Drawing for the job (mm, zero at the part's lowest x, y, z). A direction names the side the tool comes from. Give positions to 0.01 mm unless a question says otherwise; leave off trailing zeros. Order: outer loops, then holes, each group sorted by start corner. A loop starts at its lowest first (then second) coordinate and runs counter-clockwise, first axis right, second up. Notation, with made-up numbers: M 69.5,56.5 L 79.5,56.5 A23 cw 79.5,92.5 Z; hole C 4.5,35 d5. An arc over 180 degrees is marked long. Answer as a JSON object with one key per item and string values.
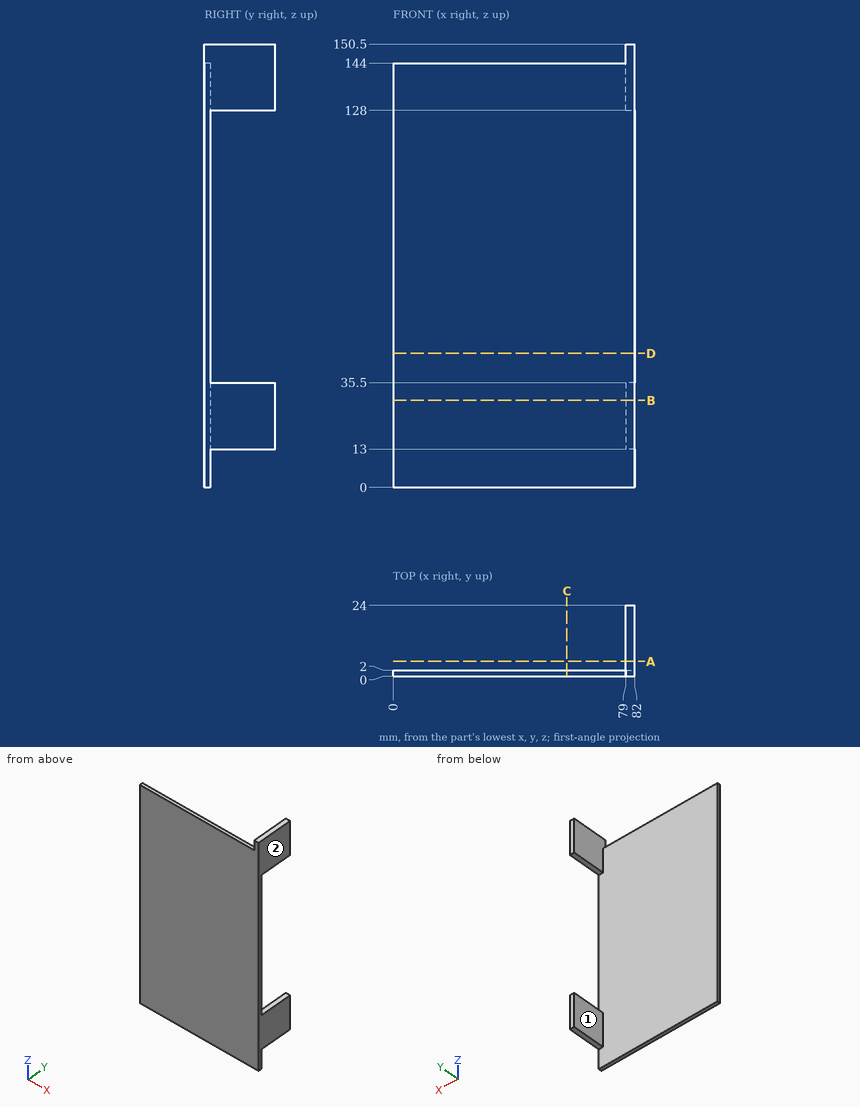
1. Which spindle directions (+Z, -Z, +X, -X, +Y, -Y) get a long thin tool onto all of the face, cutting with end or side? Do the marked faces 1 and 2. Say none if no direction does.
Worked answers:
{"face 1": "+Z, -Z, -X, +Y", "face 2": "+Z, -Z, +X, +Y, -Y"}
2. Pin check, flat tips, straight feed: P1, Ø6.5, axis at y = 12.5, z = 26.5, coming from the -X side; P2, Ø2.5, axis at x = 80, y = 11, coming from the -Z side; P3, Ø4, axis at x = 30.5, z = 80, coming from the +Y side. Stop position of each tip, or through.
Worked answers:
{"P1": "stops at x = 79", "P2": "stops at z = 13", "P3": "stops at y = 2"}
3. Cut at B-B on z = 29.5. Give the cut face in (x, y).
Worked answers:
{"outline": "M 0,0 L 82,0 L 82,24 L 79,24 L 79,2 L 0,2 Z"}
4. Cut at D-D on z = 45.5. Give the cut face in (x, y).
Worked answers:
{"outline": "M 0,0 L 82,0 L 82,2 L 0,2 Z"}
5. Cut at C-C on x = 59. Give the cut face in (y, z), plus the area to 3 significant figures.
Worked answers:
{"outline": "M 0,0 L 2,0 L 2,144 L 0,144 Z", "area": "288 mm^2"}
6. Cut at A-A on y = 5. Give the cut face in (x, z), plus the area to 3 significant figures.
Worked answers:
{"outline": "M 79,13 L 82,13 L 82,35.5 L 79,35.5 Z; M 79,128 L 82,128 L 82,150.5 L 79,150.5 Z", "area": "135 mm^2"}
7. Probe line 1 along Y through (x, z) = (16, 78); line 2 along X through (y, z) = (9.25, 130). List the from-to ranges inside material, lowest first.
Worked answers:
{"line 1": "y = 0 to 2", "line 2": "x = 79 to 82"}
